Build history of the part. All positions in model axes, mm. A direction names the side the tool comes from. Coordinates: 2 decimals unless noted, no trailing zeros. Loops run counter-clockwise (first coordinate to the right, second up) from the corner with the lowest first, then second, coordinate; pieces in that order, holes last. Notation, with made-up numbers: (-21.75, -28) - (-12.75, -28) arc R9 cw to (-12.75, -23) - close; hole circle Ø10 at (-33, -24.75). An arc over 180 degrees is marked (long way). One line per item, written item: value.
```python
from build123d import *

# Parameters (mm, degrees)
SKETCH1_W                   = 50
SKETCH1_H                   = 60
BOSS_EXTRUDE1_DEPTH         = 85.4
SKETCH2_R                   = 20.85
SKETCH2_R_2                 = 18.85
BOSS_EXTRUDE2_DEPTH         = 4.3
F_1_4_20_TAPPED_HOLE1_D     = 5.1054
F_1_4_20_TAPPED_HOLE1_DEPTH = 10.16
F_1_4_20_TAPPED_HOLE1_TIP   = 1.533816902


with BuildPart() as part:
    # Sketch1 → Boss-Extrude1 (new body)
    with BuildSketch(Plane.XY):
        Rectangle(SKETCH1_W, SKETCH1_H)
    extrude(amount=BOSS_EXTRUDE1_DEPTH)

    # Sketch2 → Boss-Extrude2 (add)
    with BuildSketch(Plane.XY.offset(85.4)):
        with Locations(Location((0, 0, 0), (0, 0, 180))):
            Circle(SKETCH2_R)
        with Locations(Location((0, 0, 0), (0, 0, 180))):
            Circle(SKETCH2_R_2, mode=Mode.SUBTRACT)
    extrude(amount=BOSS_EXTRUDE2_DEPTH)

    # 1/4-20 Tapped Hole1
    with Locations(Plane(origin=(0, -30, 0), x_dir=(-1, 0, 0), z_dir=(0, -1, 0))):
        with Locations((0, -67.85)):
            Hole(F_1_4_20_TAPPED_HOLE1_D / 2, depth=F_1_4_20_TAPPED_HOLE1_DEPTH)
            with Locations((0, 0, -(F_1_4_20_TAPPED_HOLE1_DEPTH + F_1_4_20_TAPPED_HOLE1_TIP / 2))):  # 118° drill point
                Cone(0, F_1_4_20_TAPPED_HOLE1_D / 2, F_1_4_20_TAPPED_HOLE1_TIP, mode=Mode.SUBTRACT)


solid = part.part
```
Item 1: Probe probe 1 along X at (y, z) = (-25.5, 67.85); probe 2 along Z at (x, y) = (0, -26.75); probe 3 along Y at (x, z) = (0, 87.7). List the from-to ranges inside material, lowest first. Write a range as from..to.
Check result:
probe 1: x = -25..-2.55, 2.55..25
probe 2: z = 0..65.3, 70.4..85.4
probe 3: y = -20.85..-18.85, 18.85..20.85
Item 2: Drop flat-ended pins along their axis: P1, Ø2, axis at x = -19, y = -16, coming from the -Z side; P2, Ø22.5, axis at x = 0, y = 0, coming from the +Z side; P3, Ø4, axis at x = 0, z = 67.85, coming from the -Y side. Give the stop position or say it passes through.
Check result:
P1: stops at z = 0
P2: stops at z = 85.4
P3: stops at y = -19.51
Item 3: Cut at A-A, the plane y = 0. Write the cut outline in (x, z).
Check result:
outline: (-25, 0) - (25, 0) - (25, 85.4) - (20.85, 85.4) - (20.85, 89.7) - (18.85, 89.7) - (18.85, 85.4) - (-18.85, 85.4) - (-18.85, 89.7) - (-20.85, 89.7) - (-20.85, 85.4) - (-25, 85.4) - close
Item 4: Tool access for faces 1 (the face through (0, 0, 85.4)), 2 (the face through (0, 0, 0)): list every direction of +Z, -Z, +X, -X, +Y, -Y with a clear straight run to the whole face (end or side of a thin tool).
Check result:
face 1: +Z
face 2: -Z, +X, -X, +Y, -Y
Item 5: Cut at B-B, the plane x = 6.5. Write the cut outline in (y, z), then the cut area to 3 significant figures.
Check result:
outline: (-30, 0) - (30, 0) - (30, 85.4) - (19.81, 85.4) - (19.81, 89.7) - (17.69, 89.7) - (17.69, 85.4) - (-17.69, 85.4) - (-17.69, 89.7) - (-19.81, 89.7) - (-19.81, 85.4) - (-30, 85.4) - close
area: 5,140 mm^2
Item 6: Pull direction Z, two halves, no side cores. Call faces 3 (the face through (0.1, -18.57, 68.28)), 4 (the face through (0, 30, 42)), 5 (the face through (-0.33, -24.85, 65.32)), 6 (the face through (-5.9, 20.4, 85.4)): released by +Z, released by -Z, zero draft, split by the parting line, or undercut.
Check result:
face 3: undercut
face 4: zero draft
face 5: undercut
face 6: released by +Z
